Read the model definition and answer for the solid it produces. Units are mm, in the model's axes. A direction names the side the tool comes from. Coordinates: 2 decimals unless noted, no trailing zeros. Write each loop counter-clockwise with the first axis right and the second up, starting at its lowest first coordinate (ties: lowest second). Pieces come first, ordered by that corner, then holes.
Item 1: Section D-D (x = 6) is taken. Give the vertices of the cut face in (y, z).
Item 2: Section B-B (z = 4) is taken. Give the vertices of the cut face in (x, y), then the cut area to 3 significant figures.
Item 3: Each of these flat-tipped pins is pushed along its axis until it touches: P1, Ø4, axis at x = 5, z = 7, coming from the +Y side; P2, Ø4, axis at y = 31, z = 3.5, coming from the -X side; P3, Ø2.5, axis at y = 17.5, z = 3.5, coming from the +X side. Where does it stop, or does it pass through?
Item 4: Straight lines are drawn through the part: probe 1 along Z at (x, y) = (-5.65, 41.35); probe 2 along X at (y, z) = (22.5, 6.5); probe 3 along Y at (x, z) = (8.5, 5). For each, find the intervals that lie inside material, in ascending order.
Item 5: A tool of negligible diameter and unlimited length cuts with its end or side. For faces 4 (the face through (0, 21, 4)), 5 (the face through (1, 23, 0)), 6 (the face through (8.3, 3, 4.8)), from which of +Z, -Z, +X, -X, +Y, -Y can it reach the whole face along a straight path? Write none if from no direction.
Item 6: Determine the mould class of faces 1 (the face through (-8.85, 41, 4)), 2 (the face through (5, 2, 4)), 3 (the face through (1, 23, 8)) for opening direction Z: released by +Z, released by -Z, zero draft, split by the parting line, or undercut.
Item 7: Section A-A (x = -5.65) is taken. Give the vertices of the cut face in (y, z), then the cut area to 3 significant figures.
Item 8: Section C-C (z = 6.25) is taken. Give the vertices of the cut face in (x, y), then the cut area to 3 significant figures.
Autodesk Inventor part; units mm, degrees
ref_plane "YZ Plane" through (0, 0, 0) normal (1, 0, 0) x (0, 1, 0)
ref_plane "XZ Plane" through (0, 0, 0) normal (0, 1, 0) x (-1, 0, 0)
ref_plane "XY Plane" through (0, 0, 0) normal (0, 0, 1) x (1, 0, 0)
sketch "Sketch1" plane through (0, 0, 0) normal (0, 0, 1) x (1, 0, 0)
  line L0 (0, 0) -> (3.4, 0)
  line L1 (3.4, 0) -> (3.4, 40)
  line L2 (3.4, 40) -> (0, 40)
  line L3 (0, 40) -> (0, 0)
  line L4 (3.4, 40) -> (-8.85, 40)
  line L5 (-8.85, 40) -> (-8.85, 43)
  line L6 (-8.85, 43) -> (3.4, 43)
  line L7 (3.4, 43) -> (3.4, 40)
  line L8 (3.4, 0) -> (12.25, 0)
  line L9 (12.25, 0) -> (12.25, 3)
  line L10 (12.25, 3) -> (3.4, 3)
  line L11 (3.4, 3) -> (3.4, 0)
  line L12 (-5.65, 43) -> (-5.65, 40) construction
  line L13 (-7.25, 43) -> (-7.25, 40) construction
  line L14 (-4.05, 40) -> (-4.05, 43) construction
  dimension "d0" = 40
  dimension "d1" = 3.4
  dimension "d3" = 5.65
  dimension "d4" = 3.2
  dimension "d5" = 1.6
  dimension "d6" = 1.6
  dimension "d7" = 3
  dimension "d8" = 3
  dimension "d9" = 12.25
  dimension "d10" = 12.25
extrude "Extrusion1" add sketch "Sketch1" along normal blind 8
sketch "Sketch2" plane through (-8.85, 43, 0) normal (0, 1, 0) x (1, 0, 0)
  line L0 (12.25, 0) -> (0, 0)
  line L1 (0, 0) -> (0, -8)
  line L2 (12.25, -8) -> (0, -8)
  line L3 (12.25, 0) -> (12.25, -8)
  line L4 (21.1, 0) -> (12.25, 0)
  line L5 (12.25, 0) -> (12.25, -8)
  line L6 (21.1, -8) -> (12.25, -8)
  line L7 (21.1, 0) -> (21.1, -8)
  circle A0 centre (3.2, -4) radius 1.6
  circle A1 centre (15.45, -4) radius 1.6
  line L8 (21.1, 0) -> (18.65, 0)
  line L9 (18.65, 0) -> (18.65, -8)
  line L10 (18.65, -8) -> (21.1, -8)
  line L11 (21.1, -8) -> (21.1, 0)
  point P0 (8.85, 0)
  dimension "d13" = 3.2
  dimension "d14" = 3.2
  dimension "d15" = 3.2
  dimension "d21" = 3.2
  dimension "d22" = 3.2
extrude "Extrusion2" cut sketch "Sketch2" against normal blind 51.5 contours L4 L7 L6 L9 | A0 | A1
fillet "Fillet1" radius 3 2 edges at (3.4, 43, 4) (0, 0, 4)
fillet "Fillet2" radius 1 2 edges at (3.4, 3, 4) (0, 40, 4)
equation "\"d5\" = 0.5 * d4"
equation "\"d6\" = d5"
equation "\"d10\" = d9"
properties part number "MotorBracket"
Established:
1. outline: (0, 0) - (3, 0) - (3, 2.52) - (0, 2.52) - close; (0, 5.48) - (3, 5.48) - (3, 8) - (0, 8) - close
2. outline: (-8.85, 40) - (-7.25, 40) - (-7.25, 43) - (-8.85, 43) - close; (-4.05, 40) - (-1, 40) arc R1 cw to (0, 39) - (0, 3) arc R3 ccw to (3, 0) - (5, 0) - (5, 3) - (4.4, 3) arc R1 cw to (3.4, 4) - (3.4, 40) arc R3 ccw to (0.4, 43) - (-4.05, 43) - close; (8.2, 0) - (9.8, 0) - (9.8, 3) - (8.2, 3) - close
2. area: 169 mm2
3. P1: stops at y = 41.5
3. P2: stops at x = 0
3. P3: stops at x = 3.4
4. probe 1: z = 0 to 2.4, 5.6 to 8
4. probe 2: x = 0 to 3.4
4. probe 3: y = 0 to 3
5. face 4: +Z, -Z, -X, -Y
5. face 5: -Z, +X, -X, +Y, -Y
5. face 6: +Z, -Z, +X, +Y
6. face 1: zero draft
6. face 2: undercut
6. face 3: released by +Z
7. outline: (40, 0) - (43, 0) - (43, 2.4) - (40, 2.4) - close; (40, 5.6) - (43, 5.6) - (43, 8) - (40, 8) - close
7. area: 14.4 mm2
8. outline: (-8.85, 40) - (-1, 40) arc R1 cw to (0, 39) - (0, 3) arc R3 ccw to (3, 0) - (9.8, 0) - (9.8, 3) - (4.4, 3) arc R1 cw to (3.4, 4) - (3.4, 40) arc R3 ccw to (0.4, 43) - (-8.85, 43) - close
8. area: 189 mm2
